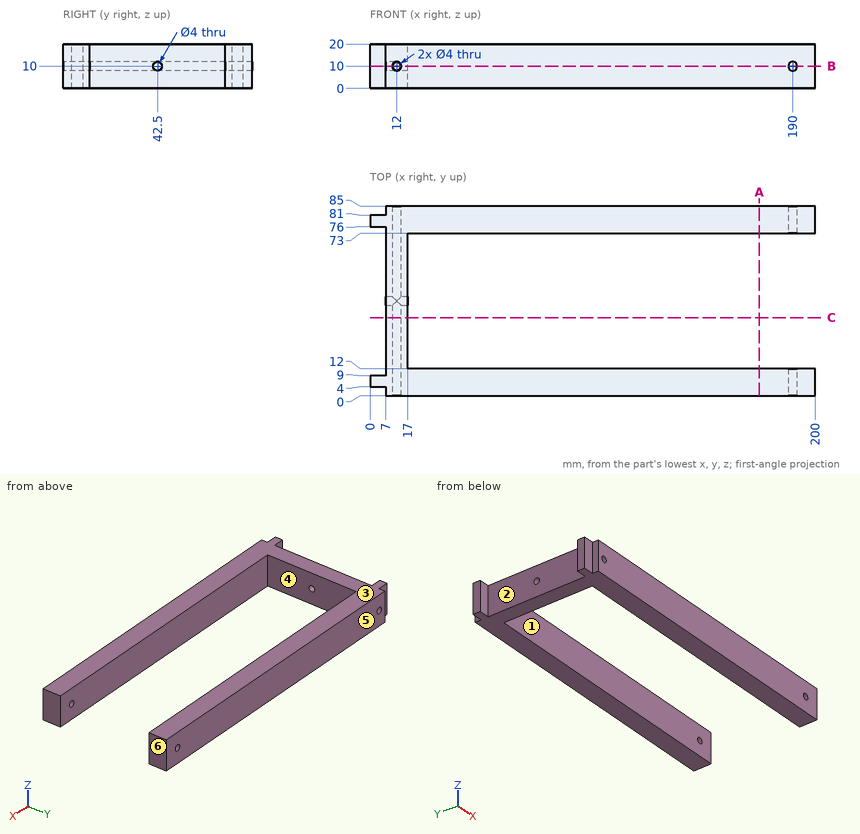
Drawing for the job (mm, zero at the part's lowest x, y, z). A direction names the side the tool comes from. Round coordinates to 2 decimals unless told otherwise and drop trailing zeros. Write each loop counter-clockwise with the first axis right and the second up, starting at its lowest first coordinate (ties: lowest second). Pieces come first, ordered by that corner, then holes. Notation, with made-up numbers: (2.5, 62) - (37.5, 62) arc R36 ccw to (37.5, 97) - close; hole circle Ø5 at (3.5, 39). An arc over 180 degrees is marked (long way). Return JSON: item names as keys, results as strings. Group by question number.
Item 1: Band-saw the part on C-C on y = 35. List the corners of the cut face in (x, z), plus the area to 3 significant figures.
Item 2: Probe probe 1 along Y at (x, z) = (28.5, 19.25); probe 2 along Y at (x, z) = (15.7, 10); probe 3 along Z at (x, y) = (14.5, 42.5). List the from-to ranges inside material, lowest first.
Item 3: Mould opens along Y. For the marked faces 4, 5 and 6 say: +Y half, -Y half, draft (parallel to the pull), parting line (faces both ways), or undercut.
Item 4: Band-saw the part on A-A on x = 175. List the corners of the cut face in (y, z), plus the area to 3 significant figures.
Item 5: 3-axis set-ups, long thin cutter, end or side, ignore diameter. For the marked faces 1, 2 and 3: which of +Z, -Z, +X, -X, +Y, -Y reach the whole face in a straight line?
Item 6: Flat gauge pins, fed straight in: pin 1 Ø7.5 at (x, z) = (3, 11.5) entering from +Y; pin 2 Ø3 at (x, z) = (12, 10) entering from +Y; pin 3 Ø2 at (y, z) = (83.5, 9) entering from -X; pin 4 Ø2 at (x, z) = (2.5, 11) entering from -Y. Where does each tip first touch, or does it go through?
Item 7: Band-saw the part on B-B on z = 10. State how many separate pieces and enclosed holes the cut face has, plus the area to 3 significant figures.
Resolved:
{
 "1": {"outline": "(7, 0) - (17, 0) - (17, 20) - (7, 20) - close; hole circle Ø4 at (12, 10)", "area": "187 mm²"},
 "2": {"probe 1": "y = 0 to 12, 73 to 85", "probe 2": "y = 0 to 40.5, 44.5 to 85", "probe 3": "z = 0 to 8, 12 to 20"},
 "3": {"face 4": "undercut", "face 5": "+Y half", "face 6": "draft"},
 "4": {"outline": "(0, 0) - (12, 0) - (12, 20) - (0, 20) - close; (73, 0) - (85, 0) - (85, 20) - (73, 20) - close", "area": "480 mm²"},
 "5": {"face 1": "+Z, -Z, +X", "face 2": "+Z, -Z, -X", "face 3": "+Z, +X, -X, +Y, -Y"},
 "6": {"pin 1": "stops at y = 81", "pin 2": "passes through", "pin 3": "stops at x = 7", "pin 4": "stops at y = 4"},
 "7": {"separate pieces": "6", "enclosed holes": "0", "area": "4,850 mm²"}
}
